Could you check a few things on this model? Use its own coordinates, in mm. Face numbers are marked on the shaded views. Give positions to 0.01 mm unless a question says otherwise; leave off trailing zeros. Write each loop counter-clockwise with the first axis right and the second up, starting at its lowest first coordinate (ties: lowest second). Pieces come first, ordered by that corner, then holes. Notation, with made-up numbers: (-9.75, 67.25) -> (29.25, 67.25) arc R15 ccw to (29.25, 71.25) -> close; hole circle Ø11 at (43.25, 65). An arc over 180 degrees is marked (long way). One line per question, with ' | ' between items.
from build123d import *

# Parameters (mm, degrees)
BOSS_EXTRUDE1_DEPTH = 7
SKETCH5_R           = 1.799999865
SKETCH5_R_2         = 1.8
CUT_EXTRUDE4_DEPTH  = 8
SKETCH2_W           = 6.5
SKETCH2_H           = 1.8
SKETCH2_H_2         = 0.9
CUT_EXTRUDE1_DEPTH  = 0.5


with BuildPart() as part:
    # Sketch1 → Boss-Extrude1 (new body)
    with BuildSketch(Plane.XY):
        with BuildLine():
            Line((9, 4), (-2.6, 4))
            ThreePointArc((-2.6, 4), (-7.1, -0.5), (-2.6, -5))
            Line((-2.6, -5), (9, -5))
            ThreePointArc((9, -5), (13.5, -0.5), (9, 4))
        make_face()
    extrude(amount=-BOSS_EXTRUDE1_DEPTH)

    # Sketch5 → Cut-Extrude4 (cut, through all)
    with BuildSketch(Plane.XY):
        with Locations((9, -0.5)):
            Circle(SKETCH5_R)
        with Locations((-2.6, -0.5)):
            Circle(SKETCH5_R_2)
    extrude(amount=-CUT_EXTRUDE4_DEPTH, mode=Mode.SUBTRACT)

    # Sketch2 → Cut-Extrude1 (cut)
    with BuildSketch(Plane.XY):
        with Locations((3.200000135, 2)):
            Rectangle(SKETCH2_W, SKETCH2_H)
        with Locations((3.200000135, -5.05)):
            Rectangle(SKETCH2_W, SKETCH2_H_2)
        with Locations((3.200000135, -0.5)):
            Rectangle(SKETCH2_W, SKETCH2_H)
        with Locations((3.200000135, -3)):
            Rectangle(SKETCH2_W, SKETCH2_H)
        with Locations((3.200000135, 4.05)):
            Rectangle(SKETCH2_W, SKETCH2_H_2)
    extrude(amount=-CUT_EXTRUDE1_DEPTH, mode=Mode.SUBTRACT)


solid = part.part
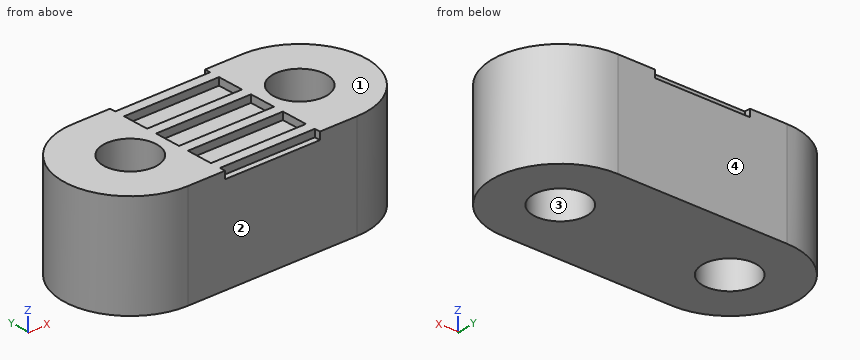
Q1. Imagine slicing it at D-D on x = 4.25. Please give me the cut outline in (y, z).
Answer below:
outline: (-5, -7) -> (4, -7) -> (4, -0.5) -> (3.6, -0.5) -> (3.6, 0) -> (2.9, 0) -> (2.9, -0.5) -> (1.1, -0.5) -> (1.1, 0) -> (0.4, 0) -> (0.4, -0.5) -> (-1.4, -0.5) -> (-1.4, 0) -> (-2.1, 0) -> (-2.1, -0.5) -> (-3.9, -0.5) -> (-3.9, 0) -> (-4.6, 0) -> (-4.6, -0.5) -> (-5, -0.5) -> close
Q2. Will these pins go through, and if not, where does the flat tip stop? pin 1 (0.6 mm diameter, centred on x = 1.5, z = 0, fed in from +Y); pin 2 (1.5 mm diameter, centred on x = 11, z = -3, fed in from +Y); pin 3 (1.5 mm diameter, centred on y = -2.5, z = -5, fed in from -X).
Answer below:
pin 1: stops at y = 3.6 | pin 2: stops at y = 3.82 | pin 3: stops at x = -6.92
Q3. If we mould it in two halves opening along Y, with no side actions, what happens to the marked faces 1, 2, 3 and 4? For each: +Y half, -Y half, draft (parallel to the pull), parting line (faces both ways), or undercut.
Answer below:
face 1: draft | face 2: -Y half | face 3: undercut | face 4: +Y half
Q4. If I drill on line 1 along Y through (x, z) = (9, -2); line 2 along X through (y, z) = (0.5, -5); line 3 along X through (y, z) = (0.25, -4), over which ranges is the centre line in solid material (lowest first)?
Answer below:
line 1: y = -5 to -2.3, 1.3 to 4 | line 2: x = -6.99 to -4.1, -1.1 to 7.5, 10.5 to 13.39 | line 3: x = -7.04 to -4.24, -0.96 to 7.36, 10.64 to 13.44
Q5. Imagine slicing it at A-A on y = -0.5. Please give me the cut outline in (x, z).
Answer below:
outline: (-7.1, -7) -> (-4.4, -7) -> (-4.4, 0) -> (-7.1, 0) -> close; (-0.8, -7) -> (7.2, -7) -> (7.2, 0) -> (6.45, 0) -> (6.45, -0.5) -> (-0.05, -0.5) -> (-0.05, 0) -> (-0.8, 0) -> close; (10.8, -7) -> (13.5, -7) -> (13.5, 0) -> (10.8, 0) -> close
Q6. Imagine slicing it at C-C on x = -2.25. Please give me the cut outline in (y, z), and give its area (3 significant figures).
Answer below:
outline: (-5, -7) -> (-2.27, -7) -> (-2.27, 0) -> (-5, 0) -> close; (1.27, -7) -> (4, -7) -> (4, 0) -> (1.27, 0) -> close | area: 38.3 mm^2
Q7. Imagine slicing it at B-B on z = -6. Please give me the cut outline in (x, y).
Answer below:
outline: (-2.6, -5) -> (9, -5) arc R4.5 ccw to (9, 4) -> (-2.6, 4) arc R4.5 ccw to start; hole circle Ø3.6 at (-2.6, -0.5); hole circle Ø3.6 at (9, -0.5)
